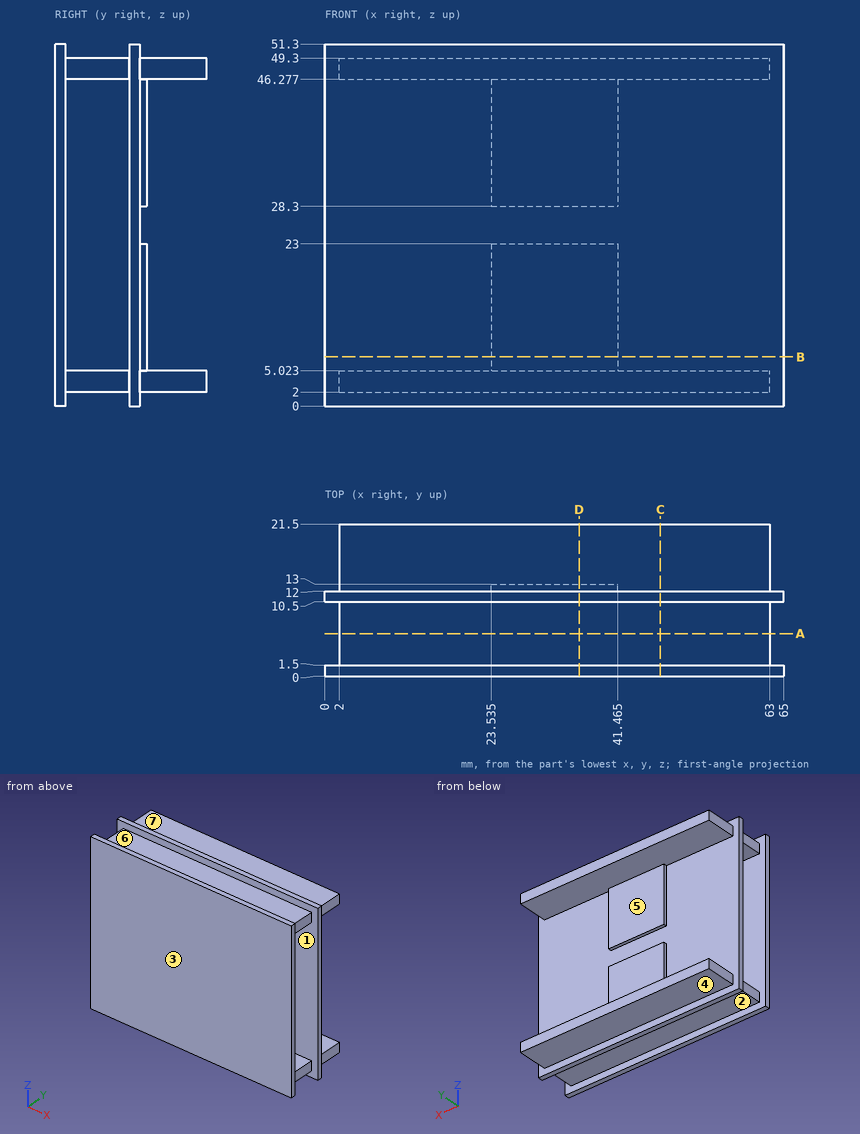
Verification items for this drawing (mm, ordinates from the low corner). A direction names the side the tool comes from. Round coordinates to 2 decimals unless told otherwise and drop trailing zeros. Loops run counter-clockwise (first coordinate to the right, second up) from the corner with the lowest first, then second, coordinate; pieces in that order, holes last. Notation, with made-up numbers: (17.5, 63.5) - (56.5, 63.5) arc R19 ccw to (56.5, 100.5) - close; hole circle Ø4 at (48.5, 49.5). An arc over 180 degrees is marked (long way). Write item = value, one per line.
Q1. Sectioned sample at D-D on x = 36. Record the boundary of the cut face in (y, z).
Here are the results:
outline = (0, 0) - (1.5, 0) - (1.5, 2) - (10.5, 2) - (10.5, 0) - (12, 0) - (12, 2) - (21.5, 2) - (21.5, 5.02) - (13, 5.02) - (13, 23) - (12, 23) - (12, 28.3) - (13, 28.3) - (13, 46.28) - (21.5, 46.28) - (21.5, 49.3) - (12, 49.3) - (12, 51.3) - (10.5, 51.3) - (10.5, 49.3) - (1.5, 49.3) - (1.5, 51.3) - (0, 51.3) - close; hole (1.5, 5.02) - (10.5, 5.02) - (10.5, 46.28) - (1.5, 46.28) - close
Q2. Sectioned sample at B-B on z = 7. Record the boundary of the cut face in (x, y) (1 decimal), plus the area to 3 significant figures.
Here are the results:
outline = (0, 0) - (65, 0) - (65, 1.5) - (0, 1.5) - close; (0, 10.5) - (65, 10.5) - (65, 12) - (41.5, 12) - (41.5, 13) - (23.5, 13) - (23.5, 12) - (0, 12) - close
area = 213 mm^2
Q3. Tool access check on the marked faces 4, 5, 6 and 7. Record the directions out of +Z, -Z, +X, -X, +Y, -Y that give a thin tool (end or side, any length) a straight path to the whole face; none if there is none.
Here are the results:
face_4 = -Z, +X, -X, +Y
face_5 = +X, -X, +Y
face_6 = +Z, +X, -X
face_7 = +Z, +X, -X, +Y
Q4. Depth check by flat-ended pin: pin 1 (2.5 mm diameter, centred on y = 4.5, z = 47.5, fed in from +X); pin 2 (5 mm diameter, centred on x = 31, y = 16, fed in from +Z); pin 3 (2.5 mm diameter, centred on x = 33.5, y = 8, fed in from -Z). Enter the tip coordinate at first touch or a pass-through.
Here are the results:
pin_1 = 63
pin_2 = 49.3
pin_3 = 2
Q5. Sectioned sample at C-C on x = 47.5. Record the boundary of the cut face in (y, z), plus the area to 3 significant figures.
Here are the results:
outline = (0, 0) - (1.5, 0) - (1.5, 2) - (10.5, 2) - (10.5, 0) - (12, 0) - (12, 2) - (21.5, 2) - (21.5, 5.02) - (12, 5.02) - (12, 46.28) - (21.5, 46.28) - (21.5, 49.3) - (12, 49.3) - (12, 51.3) - (10.5, 51.3) - (10.5, 49.3) - (1.5, 49.3) - (1.5, 51.3) - (0, 51.3) - close; hole (1.5, 5.02) - (10.5, 5.02) - (10.5, 46.28) - (1.5, 46.28) - close
area = 266 mm^2
Q6. Sectioned sample at A-A on y = 6. Record the boundary of the cut face in (x, z).
Here are the results:
outline = (2, 2) - (63, 2) - (63, 5.02) - (2, 5.02) - close; (2, 46.28) - (63, 46.28) - (63, 49.3) - (2, 49.3) - close
Q7. Mould release check, pull along Z, two halves, no side actions. Record for the marked faces 1, 2 and 3: +Z half, -Z half, draft (parallel to the pull), parting line (faces both ways), or undercut.
Here are the results:
face_1 = undercut
face_2 = -Z half
face_3 = draft
Q8. Material ranges on L1, parallel to Y at x = 27, z = 40; L2, parallel to Y at x = 42.5, z = 44; L3, parallel to Z at x = 10, y = 2.75, recorded low to high.
Here are the results:
L1 = 0 to 1.5, 10.5 to 13
L2 = 0 to 1.5, 10.5 to 12
L3 = 2 to 5.02, 46.28 to 49.3
